The listing builds one solid part. Answer for the finished solid, in the listing's coordinates (mm). A direction names the side the tool comes from. Coordinates: 2 decimals unless noted, no trailing zeros. Write each loop counter-clockwise with the first axis right and the second up, starting at its lowest first coordinate (ties: lowest second). Pieces come first, ordered by that corner, then holes.
(1) The part is cut by section B-B on z = 1. Determine the outline of the cut face in (x, y), plus the area to 3 significant figures.
(2) The part is cut by section A-A on z = 7.75. Determine the outline of the cut face in (x, y), plus the area to 3 significant figures.
(3) Straight lines are drawn through the part: line 1 (X direction, y = 0, z = 2.55); line 2 (Y direction, x = 5.5, z = 2); line 3 (Y direction, x = 0, z = 1.25). For each, find the intervals that lie inside material, in ascending order.
(4) Which of the six approach directions +Z, -Z, +X, -X, +Y, -Y give full straight-line access (tool end or side, diameter ignored) to faces 4 (the flat face through (8.9, -2, 7.5)), 5 (the cylindrical face through (0, -1, 2)), 6 (the flat face through (7, 0, 3)), 7 (the flat face through (0, -4, 6)), 8 (the flat face through (1.2, 0, 4))?
(5) For a pull along X with two mould halves and no side action, classify faces 1 (the flat face through (5.5, 4, 7)), 2 (the flat face through (8.9, 2, 7.5)), 3 (the cylindrical face through (4.25, 0.05, 1.48)) as +X half, -X half, draft (parallel to the pull), parting line (faces both ways), or undercut.
(6) The part is cut by section C-C on x = -4. Determine the outline of the cut face in (y, z).
(7) Given P1, Ø1.6, axis at y = -4, z = 7, coming from the -X side; P2, Ø1, axis at y = -1, z = 5.5, coming from the -X side; P3, Ø3.5, axis at x = 0, y = -3, coming from the +Z side; P4, Ø1.2, axis at x = 0, y = 0, coming from the -Z side, each flat-ended and moving along its own axis, determine where each tip first touches the part or whether it passes through.
(8) The part is cut by section D-D on x = 3. Determine the outline of the cut face in (y, z).
from build123d import *

# Parameters (mm, degrees)
SKETCH1_R           = 1
SKETCH1_R_2         = 1.25
BOSS_EXTRUDE1_DEPTH = 8
SKETCH2_W           = 1
SKETCH2_H           = 4
CUT_EXTRUDE1_DEPTH  = 18
CUT_EXTRUDE2_DEPTH  = 2
SKETCH4_W           = 2
SKETCH4_H           = 4
CUT_EXTRUDE3_DEPTH  = 11
SKETCH5_R           = 3
CUT_EXTRUDE4_DEPTH  = 3
SKETCH6_R           = 4
CUT_EXTRUDE5_DEPTH  = 4


with BuildPart() as part:
    # Sketch1 → Boss-Extrude1 (new body)
    with BuildSketch(Plane.XY):
        with BuildLine():
            Line((-5.5, -2), (-5.5, -5))
            Line((-5.5, -5), (5.5, -5))
            ThreePointArc((5.5, -5), (10.5, 0), (5.5, 5))
            Line((5.5, 5), (-5.5, 5))
            Line((-5.5, 5), (-5.5, 2))
            ThreePointArc((-5.5, 2), (-4.085786438, 1.414213562), (-3.5, 0))
            ThreePointArc((-3.5, 0), (-4.085786438, -1.414213562), (-5.5, -2))
        make_face()
        Circle(SKETCH1_R, mode=Mode.SUBTRACT)
        with Locations((5.5, 0)):
            Circle(SKETCH1_R_2, mode=Mode.SUBTRACT)
    extrude(amount=BOSS_EXTRUDE1_DEPTH)

    # Sketch2 → Cut-Extrude1 (cut)
    with BuildSketch(Plane.ZY.offset(5.5)):
        with Locations((7.5, 0)):
            Rectangle(SKETCH2_W, SKETCH2_H)
    extrude(amount=-CUT_EXTRUDE1_DEPTH, mode=Mode.SUBTRACT)

    # Sketch3 → Cut-Extrude2 (cut)
    with BuildSketch(Plane.XY.offset(8)):
        with BuildLine():
            Line((5.5, 3), (5.5, 5))
            Line((5.5, 5), (5.5, 6.324669678))
            Line((5.5, 6.324669678), (-9.434593506, 6.108583723))
            Line((-9.434593506, 6.108583723), (-8.586871683, -6.45764565))
            Line((-8.586871683, -6.45764565), (-0.126275451, -6.673731605))
            Line((-0.126275451, -6.673731605), (5.5, -5))
            Line((5.5, -5), (-5.5, -5))
            Line((-5.5, -5), (-5.5, -2))
            Line((-5.5, -2), (7.736067977, -2))
            ThreePointArc((7.736067977, -2), (8.238612788, 1.224744871), (5.5, 3))
        make_face()
        with BuildLine():
            ThreePointArc((5.5, -3), (6.724744871, -2.738612788), (7.736067977, -2))
            Line((7.736067977, -2), (-5.5, -2))
            Line((-5.5, -2), (-5.5, -5))
            Line((-5.5, -5), (5.5, -5))
            Line((5.5, -5), (5.5, -3))
        make_face()
    extrude(amount=-CUT_EXTRUDE2_DEPTH, mode=Mode.SUBTRACT)

    # Sketch4 → Cut-Extrude3 (cut)
    with BuildSketch(Plane.ZY.offset(5.5)):
        with Locations((5, 0)):
            Rectangle(SKETCH4_W, SKETCH4_H)
    extrude(amount=-CUT_EXTRUDE3_DEPTH, mode=Mode.SUBTRACT)

    # Sketch5 → Cut-Extrude4 (cut)
    with BuildSketch(Plane.XY.offset(6)):
        with Locations((5.5, 0)):
            Circle(SKETCH5_R)
    extrude(amount=-CUT_EXTRUDE4_DEPTH, mode=Mode.SUBTRACT)

    # Sketch6 → Cut-Extrude5 (cut)
    with BuildSketch(Plane.XY.offset(6)):
        with Locations((-5.5, 0)):
            Circle(SKETCH6_R)
    extrude(amount=-CUT_EXTRUDE5_DEPTH, mode=Mode.SUBTRACT)


solid = part.part
Model answer:
1. outline: (-5.5, -5) - (5.5, -5) arc R5 ccw to (5.5, 5) - (-5.5, 5) - (-5.5, 2) arc R2 cw to (-5.5, -2) - close; hole circle Ø2 at (0, 0); hole circle Ø2.5 at (5.5, 0)
1. area: 135 mm2
2. outline: (5.5, -5) arc R5 ccw to (10.08, -2) - (7.74, -2) arc R3 cw to (5.5, -3) - close; (5.5, 3) arc R3 cw to (7.74, 2) - (10.08, 2) arc R5 ccw to (5.5, 5) - close
2. area: 16.7 mm2
3. line 1: x = -1.5 to -1, 1 to 4.25, 6.75 to 10.5
3. line 2: y = -5 to -1.25, 1.25 to 5
3. line 3: y = -5 to -1, 1 to 5
4. face 4: +Z, +X, -X
4. face 5: +Z, -Z
4. face 6: +Z
4. face 7: +Z, -X, +Y, -Y
4. face 8: +Z, -X
5. face 1: -X half
5. face 2: draft
5. face 3: undercut
6. outline: (-5, 0) - (-1.32, 0) - (-1.32, 2) - (-3.71, 2) - (-3.71, 6) - (-5, 6) - close; (1.32, 0) - (5, 0) - (5, 6) - (3.71, 6) - (3.71, 2) - (1.32, 2) - close
7. P1: stops at x = 5.5
7. P2: stops at x = 8.1
7. P3: stops at z = 6
7. P4: passes through
8. outline: (-5, 0) - (5, 0) - (5, 6) - (2, 6) - (2, 4) - (1.66, 4) - (1.66, 3) - (-1.66, 3) - (-1.66, 4) - (-2, 4) - (-2, 6) - (-5, 6) - close
